```python
from build123d import *

# Parameters (mm, degrees)
PAD_DEPTH     = 5
SKETCH001_R   = 1.7
HOLE_DEPTH    = 72.8243
SKETCH002_W   = 30
SKETCH002_H   = 5
PAD001_DEPTH  = 5
SKETCH003_W   = 5
SKETCH003_H   = 30
PAD002_DEPTH  = 25
PAD003_DEPTH  = 5
POCKET_DEPTH  = 2.15
SKETCH006_R   = 1.7
HOLE001_DEPTH = 2.851
SKETCH007_R   = 1.9
PAD004_DEPTH  = 3.5


with BuildPart() as part:
    # Sketch → Pad (new body)
    with BuildSketch(Plane.XY):
        with BuildLine():
            Line((-15, 0), (0, 0))
            Line((0, 0), (0, 15))
            Line((0, 15), (-10, 15))
            ThreePointArc((-10, 15), (-13.535534, 13.535534), (-15, 10))
            Line((-15, 10), (-15, 0))
        make_face()
    pad = extrude(amount=PAD_DEPTH)

    # Mirrored: Pad across XZ
    add(pad.mirror(Plane.XZ))

    # Sketch001 (on Face5 of Mirrored) → Hole (cut, through all)
    with BuildSketch(Plane.XY.offset(5)):
        with Locations((-7.5, 7.5)):
            Circle(SKETCH001_R)
    hole = extrude(amount=-HOLE_DEPTH, mode=Mode.SUBTRACT)

    # Mirrored001: Hole across XZ
    add(hole.mirror(Plane.XZ), mode=Mode.SUBTRACT)

    # Sketch002 (on Face2 of Mirrored001) → Pad001 (join)
    with BuildSketch(Plane.YZ):
        with Locations((0, 2.5)):
            Rectangle(SKETCH002_W, SKETCH002_H)
    extrude(amount=PAD001_DEPTH)

    # Sketch003 (on Face12 of Pad001) → Pad002 (join)
    with BuildSketch(Plane.XY.offset(5)):
        with Locations((2.5, 0)):
            Rectangle(SKETCH003_W, SKETCH003_H)
    extrude(amount=PAD002_DEPTH)

    # Sketch004 (on Face16 of Pad002) → Pad003 (join)
    with BuildSketch(Plane.XY.offset(30)):
        with BuildLine():
            Line((5, 15), (15, 15))
            ThreePointArc((20, 10), (18.535534, 13.535534), (15, 15))
            Line((20, 10), (20, -10))
            ThreePointArc((15, -15), (18.535534, -13.535534), (20, -10))
            Line((15, -15), (5, -15))
            Line((5, -15), (5, 15))
        make_face()
    extrude(amount=-PAD003_DEPTH)

    # Sketch005 (on Face23 of Pad003) → Pocket (cut)
    with BuildSketch(Plane(origin=(0, 0, 25), x_dir=(1, 0, 0), z_dir=(0, 0, -1))):
        Polygon((15.848632, 7.5), (14.174316, 10.4), (10.825684, 10.4), (9.151368, 7.5), (10.825684, 4.6), (14.174316, 4.6), align=None)
    extrude(amount=-POCKET_DEPTH, mode=Mode.SUBTRACT)

    # Sketch006 (on Face35 of Pocket) → Hole001 (cut, through all)
    with BuildSketch(Plane(origin=(0, 0, 27.15), x_dir=(1, 0, 0), z_dir=(0, 0, -1))):
        with Locations((12.5, 7.5)):
            Circle(SKETCH006_R)
    extrude(amount=-HOLE001_DEPTH, mode=Mode.SUBTRACT)

    # Sketch007 (on Face25 of Hole001) → Pad004 (join)
    with BuildSketch(Plane.XY.offset(30)):
        with Locations((12.5, 7.5)):
            Circle(SKETCH007_R)
    extrude(amount=PAD004_DEPTH)


solid = part.part
```
Work out the finished part from the listing and answer in its coordinate system (mm). A direction names the side the tool comes from. Coordinates: 2 decimals unless noted, no trailing zeros. Write each loop counter-clockwise with the first axis right and the second up, starting at its lowest first coordinate (ties: lowest second). Pieces come first, ordered by that corner, then holes. Notation, with made-up numbers: (-7, -20) - (34, -20) arc R34 cw to (34, 14) - close; hole circle Ø9 at (81, -34.75). An arc over 180 degrees is marked (long way). Answer as a JSON object with one key per item and string values.
Q1. Given pin 1 Ø1.5 at (y, z) = (8, 21) entering from +X; pin 2 Ø4.5 at (x, y) = (-7.5, -7.5) entering from -Z; pin 3 Ø2 at (x, y) = (4, -2.5) entering from +Z; pin 4 Ø4.5 at (x, y) = (12.5, -8.5) entering from -Z, each flat-ended and moving along its own axis, determine where each tip first touches the part or whether it passes through.
Results list:
{"pin 1": "stops at x = 5", "pin 2": "stops at z = 0", "pin 3": "stops at z = 30", "pin 4": "stops at z = 25"}
Q2. Which of the six approach directions +Z, -Z, +X, -X, +Y, -Y give full straight-line access (tool end or side, diameter ignored) to faces 1 (the flat face through (0, 0, 17)), 2 (the cylindrical face through (11.1, 8.784, 31.726)), 3 (the flat face through (-15, 0, 2)), 4 (the flat face through (13, -10.4, 26))?
Results list:
{"face 1": "+Z, -X, +Y, -Y", "face 2": "+Z", "face 3": "+Z, -Z, -X, +Y, -Y", "face 4": "-Z"}
Q3. Find section D-D (y = -4). Write down the section's boundary in (x, z), plus the area to 3 significant figures.
Results list:
{"outline": "(-15, 0) - (5, 0) - (5, 25) - (20, 25) - (20, 30) - (0, 30) - (0, 5) - (-15, 5) - close", "area": "300 mm^2"}
Q4. Find section B-B (y = 7.5). Write down the section's boundary in (x, z).
Results list:
{"outline": "(-15, 0) - (-9.2, 0) - (-9.2, 5) - (-15, 5) - close; (-5.8, 0) - (5, 0) - (5, 25) - (20, 25) - (20, 30) - (14.4, 30) - (14.4, 33.5) - (10.6, 33.5) - (10.6, 30) - (0, 30) - (0, 5) - (-5.8, 5) - close"}
Q5. Find section A-A (x = -7.5). Write down the section's boundary in (y, z), plus the area to 3 significant figures.
Results list:
{"outline": "(-15, 0) - (-9.2, 0) - (-9.2, 5) - (-15, 5) - close; (-5.8, 0) - (5.8, 0) - (5.8, 5) - (-5.8, 5) - close; (9.2, 0) - (15, 0) - (15, 5) - (9.2, 5) - close", "area": "116 mm^2"}
Q6. Consider L1, parallel to Y at x = -7.5, z = 1.05; L2, parallel to Y at x = -7, z = 1; L3, parallel to Y at x = 12.5, z = 28.4. Determine where each line is inside the solid, lowest interval first. Write a range as from..to.
Results list:
{"L1": "y = -15..-9.2, -5.8..5.8, 9.2..15", "L2": "y = -15..-9.12, -5.88..5.88, 9.12..15", "L3": "y = -15..-9.2, -5.8..15"}
Q7. For a pull along Y with two mould halves and no side action, classify faces 5 (the flat face through (3, -15, 16)), 6 (the flat face through (5, 0, 12)), 7 (the flat face through (12, -4.6, 26)) as pulls with the +Y half, pulls with the -Y half, needs draft (parallel to the pull), parting line crosses it, or undercut.
Results list:
{"face 5": "pulls with the -Y half", "face 6": "needs draft", "face 7": "undercut"}
Q8. Find section C-C (x = 12.5). Write down the section's boundary in (y, z).
Results list:
{"outline": "(-15, 25) - (-10.4, 25) - (-10.4, 27.15) - (-9.2, 27.15) - (-9.2, 30) - (-15, 30) - close; (-5.8, 27.15) - (-4.6, 27.15) - (-4.6, 25) - (15, 25) - (15, 30) - (9.4, 30) - (9.4, 33.5) - (5.6, 33.5) - (5.6, 30) - (-5.8, 30) - close"}
